For this review, take the finished solid that the model builds, in its own axes (mm). Give positions to 0.01 mm unless a question says otherwise; leave off trailing zeros. Order: outer loops, then holes, each group sorted by start corner. A loop starts at its lowest first (then second) coordinate and runs counter-clockwise, first axis right, second up. Notation, with made-up numbers: M 86,7.25 L 108,7.25 A15 cw 108,18.25 Z; hole C 7.25,-1 d1. An arc over 180 degrees is marked long. Answer as CSV lines item,"result". Start each with the question number.
1. Clearance check with flat-ended pins moving along their axes: P1, Ø1.8, axis at x = 0, z = -50, coming from the -Y side; P2, Ø1.5, axis at y = 1, z = -32, coming from the +X side. State where each tip first meets the part, or that it passes through.
2. We need section A-A, the plane z = 0. Give the boundary of the cut face in (x, y), and give its area (3 significant figures).
3. For line 1 along Z through (x, y) = (-17, 1.6); line 2 along Z through (x, y) = (-40, 2.85); line 3 along X through (y, z) = (0.85, -4.5), list the stretches that pass through material, from the lowest coordinate up.
4. We need section D-D, the plane x = 30.5. Give the boundary of the cut face in (y, z), and give its area (3 significant figures).
5. Mouldability with a two-part tool opening along Z and no side actions: class faces 1 (the cylindrical face through (-48.794, 1.479, 25.379)), 2 (the cylindrical face through (36.37, 1.52, 36.46)), 3 (the flat face through (-45, 0, -8)) as pulls with the +Z half, pulls with the -Z half, needs draft (parallel to the pull), parting line crosses it, or undercut.
6. We need section B-B, the plane z = -50. Give the boundary of the cut face in (x, y), and give its area (3 significant figures).
7. We need section C-C, the plane y = 1.4. State how many separate pieces and enclosed holes the cut face has, and give its area (3 significant figures).
from build123d import *

# Parameters (mm, degrees)
SKETCH1_R           = 55
SKETCH1_R_2         = 45
BOSS_EXTRUDE1_DEPTH = 3
SKETCH3_R           = 1.5
CUT_EXTRUDE1_DEPTH  = 3
CRVPATTERN1_COUNT   = 8


with BuildPart() as part:
    # Sketch1 → Boss-Extrude1 (new body)
    with BuildSketch(Plane(origin=(0, 0, 0), x_dir=(1, 0, 0), z_dir=(0, 1, 0))):
        with Locations(Location((0, 0, 0), (0, 0, 270))):
            Circle(SKETCH1_R)
        with Locations(Location((0, 0, 0), (0, 0, 270))):
            Circle(SKETCH1_R_2, mode=Mode.SUBTRACT)
    extrude(amount=BOSS_EXTRUDE1_DEPTH)

    # Sketch3 → Cut-Extrude1 (cut)
    with BuildSketch(Plane(origin=(0, 3, 0), x_dir=(1, 0, 0), z_dir=(0, 1, 0))):
        with Locations(Location((0, 50, 0), (0, 0, 270))):
            Circle(SKETCH3_R)
    cut_extrude1 = extrude(amount=-CUT_EXTRUDE1_DEPTH, mode=Mode.SUBTRACT)

    # CrvPattern1: Cut-Extrude1 ×8 about axis
    crvpattern1_axis = Axis((0, 3, 0), (0, 1, 0))
    for i in range(1, CRVPATTERN1_COUNT):
        add(cut_extrude1.rotate(crvpattern1_axis, i * 360 / CRVPATTERN1_COUNT), mode=Mode.SUBTRACT)


solid = part.part
Result set:
1,P1,"through"
1,P2,"x = 45.26"
2,outline,"M -55,0 L -51.5,0 L -51.5,3 L -55,3 Z; M -48.5,0 L -45,0 L -45,3 L -48.5,3 Z; M 45,0 L 48.5,0 L 48.5,3 L 45,3 Z; M 51.5,0 L 55,0 L 55,3 L 51.5,3 Z"
2,area,"42.0 mm2"
3,line 1,"-52.31 to -41.67, 41.67 to 52.31"
3,line 2,"-37.75 to -20.62, 20.62 to 37.75"
3,line 3,"-54.82 to -44.77, 44.77 to 54.82"
4,outline,"M 0,-45.77 L 3,-45.77 L 3,-33.09 L 0,-33.09 Z; M 0,33.09 L 3,33.09 L 3,45.77 L 0,45.77 Z"
4,area,"76.1 mm2"
5,face 1,"parting line crosses it"
5,face 2,"undercut"
5,face 3,"needs draft"
6,outline,"M -22.91,0 L -1.5,0 L -1.5,3 L -22.91,3 Z; M 1.5,0 L 22.91,0 L 22.91,3 L 1.5,3 Z"
6,area,"128 mm2"
7,separate pieces,"1"
7,enclosed holes,"9"
7,area,"3,090 mm2"
